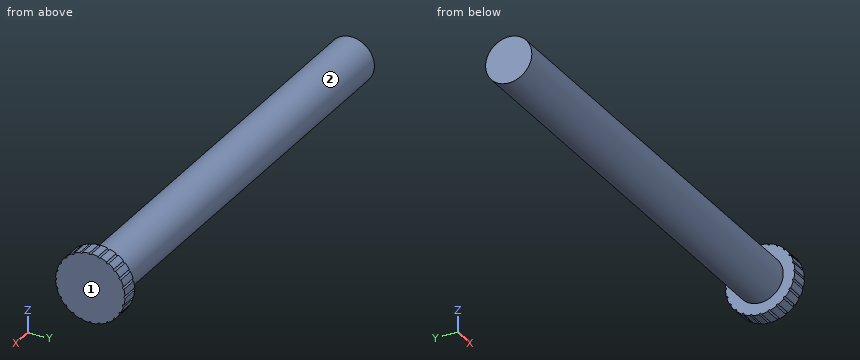
from build123d import *

# Parameters (mm, degrees)
SKETCH1_R           = 4
BOSS_EXTRUDE1_DEPTH = 78.63
SKETCH2_R           = 6
BOSS_EXTRUDE2_DEPTH = 3
SKETCH3_R           = 0.2
CUT_EXTRUDE1_DEPTH  = 3
CIRPATTERN1_COUNT   = 24


with BuildPart() as part:
    # Sketch1 → Boss-Extrude1 (new body)
    with BuildSketch(Plane(origin=(0, 0, 0), x_dir=(0, 0, -1), z_dir=(1, 0, 0))):
        Circle(SKETCH1_R)
    extrude(amount=BOSS_EXTRUDE1_DEPTH)

    # Sketch2 → Boss-Extrude2 (add)
    with BuildSketch(Plane(origin=(78.63, 0, 0), x_dir=(0, 0, -1), z_dir=(1, 0, 0))):
        Circle(SKETCH2_R)
    extrude(amount=BOSS_EXTRUDE2_DEPTH)

    # Sketch3 → Cut-Extrude1 (cut)
    with BuildSketch(Plane(origin=(81.63, 0, 0), x_dir=(0, 0, -1), z_dir=(1, 0, 0))):
        with Locations((-6, 0)):
            Circle(SKETCH3_R)
    cut_extrude1 = extrude(amount=-CUT_EXTRUDE1_DEPTH, mode=Mode.SUBTRACT)

    # CirPattern1: Cut-Extrude1 ×24 about axis
    cirpattern1_axis = Axis((0, 0, 0), (1, 0, 0))
    for i in range(1, CIRPATTERN1_COUNT):
        add(cut_extrude1.rotate(cirpattern1_axis, i * 360 / CIRPATTERN1_COUNT), mode=Mode.SUBTRACT)


solid = part.part
Can you work these out from the model? Positions are in its coordinate system, mm. Face numbers are marked on the shaded views. A direction names the side the tool comes from. Coordinates: 2 decimals unless noted, no trailing zeros. Loops run counter-clockwise (first coordinate to the right, second up) from the corner with the lowest first, then second, coordinate; pieces in that order, holes last. Notation, with made-up numbers: M -7,12 L 6,12 A34 ccw 6,49 Z; hole C 73.25,-28.75 d8. An arc over 180 degrees is marked long. Answer as CSV lines item,"result". Start each with the question number.
1. For the marked faces 1 and 2, which set-ups out of +Z, -Z, +X, -X, +Y, -Y let a thin tool reach every point of the face, with its end or its side?
2. If I drill on probe 1 along X at (y, z) = (0.75, -5); probe 2 along Y at (x, z) = (28, 0); probe 3 along Z at (x, y) = (53.5, 2), over which ranges is the centre line in solid material (lowest first)? Write a range as [from, to].
3. For pin 1 Ø6 at (x, z) = (72, 5) entering from -Y; pin 2 Ø2 at (x, z) = (67, -1.5) entering from +Y; pin 3 Ø3 at (x, y) = (44, 4.5) entering from +Z, each with a flat end and sliding along its axis, tell me the tip position at first contact or that it passes through.
4. Suppose I cut it at A-A, the plane x = 21. List the corners of the cut face in (y, z) for me, plus the area to 3 significant figures.
Output:
1,face 1,"+Z, -Z, +X, +Y, -Y"
1,face 2,"-X"
2,probe 1,"x = [78.63, 81.63]"
2,probe 2,"y = [-4, 4]"
2,probe 3,"z = [-3.46, 3.46]"
3,pin 1,"stops at y = -3.46"
3,pin 2,"stops at y = 3.97"
3,pin 3,"stops at z = 2.65"
4,outline,"C 0,0 d8"
4,area,"50.3 mm^2"
